from build123d import *

# Parameters (mm, degrees)
F0_R     = 3
F1_DEPTH = 5


with BuildPart() as f1:
    # F0 (on Front) → F1 (new body)
    with BuildSketch(Plane.XZ):
        with BuildLine():
            Line((42.073386, 42.901178), (-42.073386, 42.901178))
            ThreePointArc((-42.073386, 42.901178), (-47.208268, 40.004884), (-47.385773, 34.112174))
            Line((-47.385773, 34.112174), (-11.685773, -33.887826))
            ThreePointArc((-11.685773, -33.887826), (0, -41.72783), (11.685773, -33.887826))
            Line((11.685773, -33.887826), (47.385773, 34.112174))
            ThreePointArc((47.385773, 34.112174), (47.208268, 40.004884), (42.073386, 42.901178))
        make_face()
        with Locations((0, -29.098822)):
            Circle(F0_R, mode=Mode.SUBTRACT)
        with BuildLine():
            Line((-9.620267, -20.611675), (-35.688363, 29.041842))
            ThreePointArc((-35.688363, 29.041842), (-35.570026, 32.970315), (-32.146772, 34.901178))
            Line((-32.146772, 34.901178), (32.146772, 34.901178))
            ThreePointArc((32.146772, 34.901178), (35.570026, 32.970315), (35.688363, 29.041842))
            Line((35.688363, 29.041842), (9.620267, -20.611675))
            ThreePointArc((9.620267, -20.611675), (7.176721, -22.598675), (4.05245, -22.201167))
            ThreePointArc((4.05245, -22.201167), (0, -21.098822), (-4.05245, -22.201167))
            ThreePointArc((-4.05245, -22.201167), (-7.176721, -22.598675), (-9.620267, -20.611675))
        make_face(mode=Mode.SUBTRACT)
    extrude(amount=F1_DEPTH)


solid = f1.part
The listing builds one solid part. Answer for the finished solid, in the listing's coordinates (mm). A direction names the side the tool comes from. Give positions to 0.01 mm unless a question says otherwise; leave off trailing zeros. Order: outer loops, then holes, each group sorted by start corner. A loop starts at its lowest first (then second) coordinate and runs counter-clockwise, first axis right, second up. Notation, with made-up numbers: (-30.5, 61.5) - (-15.5, 61.5) arc R18 cw to (-15.5, 86.5) - close; hole circle Ø4 at (22, -33). An arc over 180 degrees is marked (long way). One line per item, written item: value. Start each with the question number.
1) The mould has two halves that part along X. Classify faces 3 (the face through (29.29, -2.46, -0.36)), 4 (the face through (-0.209, -2.465, -41.726)), 5 (the face through (-7.13, -2.46, -22.61)): released by +X, released by -X, zero draft, split by the parting line, or undercut.
2) A cutting plane is placed at A-A on x = 0. Give the vertices of the cut face in (y, z).
3) A cutting plane is placed at B-B on z = 33. Give the vertices of the cut face in (x, y), then the cut area to 4 significant figures.
4) A cutting plane is placed at C-C on y = -1.65. Give the vertices of the cut face in (x, z), then the cut area to 3 significant figures.
5) A tool of negligible diameter and unlimited length cuts with its end or side. For faces 1 (the face through (47.252, -2.465, 39.931)), 2 (the face through (-35.6, -2.46, 32.92)), from which of +Z, -Z, +X, -X, +Y, -Y can it reach the whole face along a straight path? Write none if from no direction.
6) Find the intervals of material crossed by L1, parallel to X at y = -2.9, z = 8.5; L2, parallel to X at y = -1.3, z = 14; L3, parallel to Z at x = -22.5, y = -2.05, in increasing order.
7) Given pin 1 Ø9.5 at (x, z) = (0, -29.1) entering from -Y; pin 2 Ø1.5 at (y, z) = (-4.5, -2.5) entering from +X, each flat-ended and moving along its own axis, determine where each tip first touches the part or whether it passes through.
Answer sheet:
1. face 3: released by +X
1. face 4: split by the parting line
1. face 5: undercut
2. outline: (-5, -41.73) - (0, -41.73) - (0, -32.1) - (-5, -32.1) - close; (-5, -26.1) - (0, -26.1) - (0, -21.1) - (-5, -21.1) - close; (-5, 34.9) - (0, 34.9) - (0, 42.9) - (-5, 42.9) - close
3. outline: (-46.8, -5) - (-35.55, -5) - (-35.55, 0) - (-46.8, 0) - close; (35.55, -5) - (46.8, -5) - (46.8, 0) - (35.55, 0) - close
3. area: 112.5 mm2
4. outline: (-47.39, 34.11) - (-11.69, -33.89) arc R12.63 ccw to (11.69, -33.89) - (47.39, 34.11) arc R6 ccw to (42.07, 42.9) - (-42.07, 42.9) arc R6 ccw to start; hole (-35.69, 29.04) - (-9.62, -20.61) arc R4 ccw to (-4.05, -22.2) arc R8 cw to (4.05, -22.2) arc R4 ccw to (9.62, -20.61) - (35.69, 29.04) arc R4 ccw to (32.15, 34.9) - (-32.15, 34.9) arc R4 ccw to start; hole circle Ø6 at (0, -29.1)
4. area: 2,260 mm2
5. face 1: +X, +Y, -Y
5. face 2: +Y, -Y
6. L1: x = -33.94 to -24.9, 24.9 to 33.94
6. L2: x = -36.83 to -27.79, 27.79 to 36.83
6. L3: z = -13.29 to 3.92, 34.9 to 42.9
7. pin 1: stops at y = -5
7. pin 2: stops at x = 28.56
